CAD build for the part. Positions are in the model's coordinates, mm. Give positions to 0.01 mm unless a question says otherwise; leave off trailing zeros. Order: outer loops, then holes, each group sorted by start corner. A loop starts at its lowest first (then second) coordinate and runs counter-clockwise, first axis right, second up.
from build123d import *

# Parameters (mm, degrees)
SKETCH1_W           = 292.1
SKETCH1_H           = 158.75
BOSS_EXTRUDE1_DEPTH = 6.35
SKETCH2_R           = 3.175
CUT_EXTRUDE2_DEPTH  = 6.35
SKETCH4_R           = 1.5875
CUT_EXTRUDE3_DEPTH  = 7.35
SKETCH5_R           = 1.525
CUT_EXTRUDE4_DEPTH  = 7.35


with BuildPart() as part:
    # Sketch1 → Boss-Extrude1 (new body)
    with BuildSketch(Plane(origin=(0, 0, 0), x_dir=(1, 0, 0), z_dir=(0, 1, 0))):
        with Locations((146.05, 79.375)):
            Rectangle(SKETCH1_W, SKETCH1_H)
    extrude(amount=BOSS_EXTRUDE1_DEPTH)

    # Sketch2 → Cut-Extrude2 (cut)
    with BuildSketch(Plane(origin=(0, 6.35, 0), x_dir=(1, 0, 0), z_dir=(0, 1, 0))):
        with Locations((146.05, 12.7)):
            Circle(SKETCH2_R)
        with Locations((247.65, 12.7)):
            Circle(SKETCH2_R)
        with Locations((44.45, 12.7)):
            Circle(SKETCH2_R)
    extrude(amount=-CUT_EXTRUDE2_DEPTH, mode=Mode.SUBTRACT)

    # Sketch4 → Cut-Extrude3 (cut, through all)
    with BuildSketch(Plane(origin=(0, 6.35, 0), x_dir=(1, 0, 0), z_dir=(0, 1, 0))):
        with Locations((182.88, 82.55)):
            Circle(SKETCH4_R)
        with Locations((189.23, 34.29)):
            Circle(SKETCH4_R)
        with Locations((265.43, 82.55)):
            Circle(SKETCH4_R)
        with Locations((264.16, 34.29)):
            Circle(SKETCH4_R)
        with Locations((264.795, 142.875)):
            Circle(SKETCH4_R)
        with Locations((264.795, 94.615)):
            Circle(SKETCH4_R)
        with Locations((198.755, 97.79)):
            Circle(SKETCH4_R)
        with Locations((198.755, 139.7)):
            Circle(SKETCH4_R)
        with Locations((102.87, 82.55)):
            Circle(SKETCH4_R)
        with Locations((109.22, 34.29)):
            Circle(SKETCH4_R)
        with Locations((26.67, 34.29)):
            Circle(SKETCH4_R)
        with Locations((27.94, 82.55)):
            Circle(SKETCH4_R)
        with Locations((93.345, 139.7)):
            Circle(SKETCH4_R)
        with Locations((93.345, 97.79)):
            Circle(SKETCH4_R)
        with Locations((27.305, 142.875)):
            Circle(SKETCH4_R)
        with Locations((27.305, 94.615)):
            Circle(SKETCH4_R)
    extrude(amount=-CUT_EXTRUDE3_DEPTH, mode=Mode.SUBTRACT)

    # Sketch5 → Cut-Extrude4 (cut, through all)
    with BuildSketch(Plane(origin=(0, 6.35, 0), x_dir=(1, 0, 0), z_dir=(0, 1, 0))):
        with Locations((279.4, 31.75)):
            Circle(SKETCH5_R)
        with Locations((279.4, 75.25)):
            Circle(SKETCH5_R)
        with Locations((143.9, 75.25)):
            Circle(SKETCH5_R)
        with Locations((143.9, 31.75)):
            Circle(SKETCH5_R)
    extrude(amount=-CUT_EXTRUDE4_DEPTH, mode=Mode.SUBTRACT)


solid = part.part
1. Saw through at B-B on x = 247.65. Give the cut face in (y, z) (3 decimals).
2. Wall check: line 1 (X direction, y = 2.75, z = -32); line 2 (Z direction, x = 146, y = 3); line 3 (Z direction, x = 182.88, y = 1.75). Give the ranges that are in metal, low to high.
3. Saw through at A-A on z = -12.7. Give the cut face in (x, y) (3 decimals).
4. Mould opens along Z. For faces 1 (the cylindrical face through (148.98, 3.22, -11.48)), 2 (the flat face through (144, 3, 0)), 3 (the flat face through (144, 0, -80)) say: released by +Z, released by -Z, zero draft, split by the parting line, or undercut.
5. Pin check, flat tip, straight feed: P1, Ø3, axis at x = 198.755, z = -97.79, coming from the -Y side. Stop position of the tip, or through.
Reported:
1. outline: (0, -158.75) - (6.35, -158.75) - (6.35, -15.875) - (0, -15.875) - close; (0, -9.525) - (6.35, -9.525) - (6.35, 0) - (0, 0) - close
2. line 1: x = 0 to 142.4, 145.4 to 277.9, 280.9 to 292.1
2. line 2: z = -158.75 to -15.87, -9.53 to 0
2. line 3: z = -158.75 to -84.14, -80.96 to 0
3. outline: (0, 0) - (41.275, 0) - (41.275, 6.35) - (0, 6.35) - close; (47.625, 0) - (142.875, 0) - (142.875, 6.35) - (47.625, 6.35) - close; (149.225, 0) - (244.475, 0) - (244.475, 6.35) - (149.225, 6.35) - close; (250.825, 0) - (292.1, 0) - (292.1, 6.35) - (250.825, 6.35) - close
4. face 1: undercut
4. face 2: released by +Z
4. face 3: zero draft
5. P1: passes through
